For this review, take the finished solid that the model builds, in its own axes (mm). A direction names the side the tool comes from. Coordinates: 2 decimals unless noted, no trailing zeros. Order: outer loops, then holes, each group sorted by start corner. A loop starts at its lowest first (then second) coordinate and runs counter-clockwise, first axis right, second up. Notation, with made-up numbers: M 67.25,47 L 103.25,47 A13 cw 103.25,58 Z; hole C 19.25,21 d8. An arc over 180 degrees is marked long. Use one line per item in the form item = value. Start each with the question number.
```python
from build123d import *

# Parameters (mm, degrees)
BOSS_EXTRUDE1_DEPTH = 50.8
CUT_EXTRUDE1_DEPTH  = 2.27


with BuildPart() as part:
    # Sketch2 → Boss-Extrude1 (new body, symmetric)
    with BuildSketch(Plane(origin=(0, 0, 0), x_dir=(1, 0, 0), z_dir=(0, 1, 0))):
        with BuildLine():
            Line((0.381, 0), (20.066, 0))
            ThreePointArc((20.066, 0), (20.335407684, -0.111592316), (20.447, -0.381))
            Line((20.447, -0.381), (20.447, -0.889))
            ThreePointArc((20.447, -0.889), (20.335407684, -1.158407684), (20.066, -1.27))
            Line((20.066, -1.27), (1.651, -1.27))
            ThreePointArc((1.651, -1.27), (1.381592316, -1.381592316), (1.27, -1.651))
            Line((1.27, -1.651), (1.27, -3.937))
            ThreePointArc((1.27, -3.937), (1.381592316, -4.206407684), (1.651, -4.318))
            Line((1.651, -4.318), (2.03996875, -4.318))
            ThreePointArc((2.03996875, -4.318), (2.174672592, -4.293392866), (2.291976563, -4.22275))
            ThreePointArc((2.291976563, -4.22275), (4.191, -5.08), (2.291976563, -5.93725))
            ThreePointArc((2.291976563, -5.93725), (2.174672592, -5.866607134), (2.03996875, -5.842))
            Line((2.03996875, -5.842), (0.381, -5.842))
            ThreePointArc((0.381, -5.842), (0.111592316, -5.730407684), (0, -5.461))
            Line((0, -5.461), (0, -0.381))
            ThreePointArc((0, -0.381), (0.111592316, -0.111592316), (0.381, 0))
        make_face()
    extrude(amount=BOSS_EXTRUDE1_DEPTH, both=True)

    # Sketch7 → Cut-Extrude1 (cut, through all)
    with BuildSketch(Plane.XY.offset(1.27)):
        with BuildLine():
            Line((11.71575, 2.38125), (13.30325, 2.38125))
            ThreePointArc((13.30325, 2.38125), (15.6845, 0), (13.30325, -2.38125))
            Line((13.30325, -2.38125), (11.71575, -2.38125))
            ThreePointArc((11.71575, -2.38125), (9.3345, 0), (11.71575, 2.38125))
        make_face()
    extrude(amount=-CUT_EXTRUDE1_DEPTH, mode=Mode.SUBTRACT)


solid = part.part
```
1. For pin 1 Ø3 at (y, z) = (24.5, 4.5) entering from +X; pin 2 Ø1.8 at (y, z) = (25, 2.5) entering from +X; pin 3 Ø1 at (x, z) = (15, 3.5) entering from -Y; pin 4 Ø0.5 at (x, y) = (1, -25) entering from +Z, all flat-tipped, find the tip position at first contact; note any pin that passes through.
2. To check wall thickness, follow line 1 (X direction, y = -26.5, z = 3.25); line 2 (X direction, y = -13, z = 1). State the ranges of each line that lie inside material, in increasing order.
3. The part is to be moulded in two halves that separate along Y. For faces 1 (the flat face through (8, 50.8, 1)), 2 (the flat face through (1.27, 1, 3)), 3 (the cylindrical face through (9.335, -0.052, 0.644)), 4 (the cylindrical face through (15.684, 0.052, 0.644)), say which applies: pulls with the +Y half, pulls with the -Y half, needs draft (parallel to the pull), parting line crosses it, or undercut.
4. Consider section B-B, the plane x = 14.75. Write out the cut boundary in (y, z), plus the area to 3 significant figures.
5. Consider section A-A, the plane y = 0. Write out the cut boundary in (x, z), plus the area to 3 significant figures.
6. Consider section C-C, the plane y = -36. Write out the cut boundary in (x, z), plus the area to 3 significant figures.
7. Consider section D-D, the plane z = 2.5. Write out the cut boundary in (x, y).
8. Tool access review of faces 5 (the flat face through (8, -50.8, 1)), 6 (the flat face through (1, 1, 5.842)): name each direction out of +Z, -Z, +X, -X, +Y, -Y from which nothing blocks a thin tool from reaching the whole face with its end or side.
Answers follow:
q1.pin_1 = 4.19
q1.pin_2 = 1.27
q1.pin_3 = through
q1.pin_4 = 5.84
q2.line_1 = 0 to 1.27
q2.line_2 = 0 to 20.43
q3.face_1 = pulls with the +Y half
q3.face_2 = needs draft
q3.face_3 = undercut
q3.face_4 = undercut
q4.outline = M -50.8,0 L -1.89,0 L -1.89,1.27 L -50.8,1.27 Z; M 1.89,0 L 50.8,0 L 50.8,1.27 L 1.89,1.27 Z
q4.area = 124 mm²
q5.outline = M 0,0.38 A0.38 ccw 0.38,0 L 9.33,0 L 9.33,1.27 L 1.65,1.27 A0.38 cw 1.27,1.65 L 1.27,3.94 A0.38 cw 1.65,4.32 L 2.04,4.32 A0.38 cw 2.29,4.22 A1.14 ccw long 2.29,5.94 A0.38 cw 2.04,5.84 L 0.38,5.84 A0.38 ccw 0,5.46 Z; M 15.68,0 L 20.07,0 A0.38 ccw 20.45,0.38 L 20.45,0.89 A0.38 ccw 20.07,1.27 L 15.68,1.27 Z
q5.area = 28.9 mm²
q6.outline = M 0,0.38 A0.38 ccw 0.38,0 L 20.07,0 A0.38 ccw 20.45,0.38 L 20.45,0.89 A0.38 ccw 20.07,1.27 L 1.65,1.27 A0.38 cw 1.27,1.65 L 1.27,3.94 A0.38 cw 1.65,4.32 L 2.04,4.32 A0.38 cw 2.29,4.22 A1.14 ccw long 2.29,5.94 A0.38 cw 2.04,5.84 L 0.38,5.84 A0.38 ccw 0,5.46 Z
q6.area = 36.9 mm²
q7.outline = M 0,-50.8 L 1.27,-50.8 L 1.27,50.8 L 0,50.8 Z
q8.face_5 = +Z, -Z, +X, -X, -Y
q8.face_6 = +Z, -X, +Y, -Y
